from build123d import *

# Parameters (mm, degrees)
F0_W        = 159.9819
F0_H        = 117.475
F1_DEPTH    = 18.25625
F3_D        = 7.9375
F5_D        = 7.9375
F6_T1_DEPTH = 225.3026478943
F7_T1_DEPTH = 192.6422739472


# Not quite as in the source:
# - a fillet or chamfer that OpenCascade refuses, or shapes differently, is made with other operations: its cross-section is extruded or revolved along the edge and cut away or added


with BuildPart() as f1:
    # F0 (on Top) → F1 (new body)
    with BuildSketch(Plane.XY):
        with Locations((79.99095, 58.7375)):
            Rectangle(F0_W, F0_H)
    extrude(amount=F1_DEPTH)

    # F3 (through all)
    with Locations(Plane.XY.offset(18.25625)):
        with Locations((27.90825, 12.7), (132.07365, 12.7)):
            Hole(F3_D / 2)

    # F5 (through all)
    with Locations(Plane.XY.offset(18.25625)):
        with Locations((27.90825, 111.125), (132.07365, 111.125)):
            Hole(F5_D / 2)

    # F6: chamfer of 12.7 on 1 edges, made by hand

    # F6_s2 → F6_t1 (cut)
    with BuildSketch(Plane.YZ.offset(-32.6603739472)):
        Polygon((0, 12.7), (12.7, 0), (0, 0), align=None)
    extrude(amount=F6_T1_DEPTH, mode=Mode.SUBTRACT)

    # F7: chamfer of 6.35 on 1 edges, made by hand

    # F7_s2 → F7_t1 (cut)
    with BuildSketch(Plane.YZ.offset(-16.3301869736)):
        Polygon((111.125, 0), (117.475, 6.35), (117.475, 0), align=None)
    extrude(amount=F7_T1_DEPTH, mode=Mode.SUBTRACT)


solid = f1.part
Here's how the part is built. I have some questions about the finished solid (model axes, mm). Round coordinates to 2 decimals unless told otherwise and drop trailing zeros. Loops run counter-clockwise (first coordinate to the right, second up) from the corner with the lowest first, then second, coordinate; pieces in that order, holes last. Notation, with made-up numbers: M -25.75,-22.75 L 10.25,-22.75 A20 ccw 10.25,-5.75 Z; hole C -17.5,-7 d3. An arc over 180 degrees is marked long. Write each question's results on one line, items separated by ' | '. Start each with the question number.
(1) Thinking about a two-plate mould opening in X: for faces 1 (the cylindrical face through (132.93, 107.25, 9)), 2 (the flat face through (78.871, 114.256, 3.131)), 3 (the flat face through (0, 58, 9)), which applies, pulls with the +X half, pulls with the -X half, needs draft (parallel to the pull), parting line crosses it, or undercut?
(2) I want a section at B-B (z = 2). Please give me the cut outline in (x, y) (1 decimal).
(3) If I drill on probe 1 along Y at (x, z) = (129.5, 16.5) (3 decimals); probe 2 along Y at (x, z) = (11, 11.75) (3 decimals); probe 3 along Y at (x, z) = (23, 9.5) (3 decimals), over which ranges is the centre line in solid material (lowest first)? Write a range as from..to.
(4) Will these pins go through, and if not, where does the flat tip stop? P1, Ø5, axis at x = 49, z = 3.5, coming from the -Y side; P2, Ø5, axis at x = 107, z = 5, coming from the -Y side.
(5) I want a section at A-A (x = 119). Please give me the cut outline in (y, z) (3 decimals).
Solved:
1) face 1: undercut | face 2: needs draft | face 3: pulls with the -X half
2) outline: M 0,10.7 L 24.5,10.7 A4 cw long 31.3,10.7 L 128.6,10.7 A4 cw long 135.5,10.7 L 160,10.7 L 160,113.1 L 135.5,113.1 A4 cw long 128.6,113.1 L 31.3,113.1 A4 cw long 24.5,113.1 L 0,113.1 Z
3) probe 1: y = 0..9.679, 15.721..108.104, 114.146..117.475 | probe 2: y = 0.95..117.475 | probe 3: y = 3.2..117.475
4) P1: stops at y = 6.7 | P2: stops at y = 5.2
5) outline: M 0,12.7 L 12.7,0 L 111.125,0 L 117.475,6.35 L 117.475,18.256 L 0,18.256 Z
